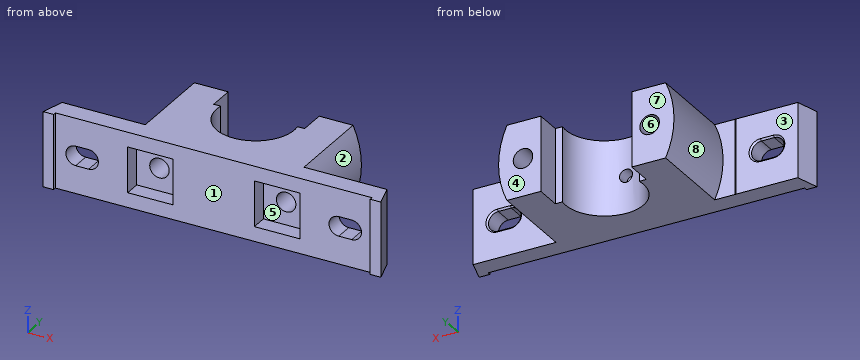
from build123d import *

# Parameters (mm, degrees)
BOSS_EXTRUDE2_DEPTH  = 46
CUT_EXTRUDE1_START   = -52.000000108
CUT_EXTRUDE1_DEPTH   = 36.000000108
CUT_EXTRUDE1_START_2 = 18
CUT_EXTRUDE1_2_DEPTH = 10
CUT_EXTRUDE4_DEPTH   = 126.888839891
CHAMFER1_SIZE        = 1
CUT_EXTRUDE6_DEPTH   = 54
SKETCH7_W            = 28
SKETCH7_H            = 28
CUT_EXTRUDE7_DEPTH   = 10
SKETCH8_R            = 6
CUT_EXTRUDE8_DEPTH   = 127.759615321


with BuildPart() as part:
    # Sketch1 → Boss-Extrude2 (new body)
    with BuildSketch(Plane.XY):
        with BuildLine():
            Line((-28, 20), (-28, 4))
            Line((-28, 4), (-23.664319132, 4))
            ThreePointArc((-23.664319132, 4), (0, -24), (23.664319132, 4))
            Line((23.664319132, 4), (28, 4))
            Line((28, 4), (28, 20))
            Line((28, 20), (54, 20))
            Line((54, 20), (54, -26))
            ThreePointArc((54, -26), (56.343145751, -31.656854249), (62, -34))
            Line((62, -34), (99.985564599, -34))
            Line((99.985564599, -34), (104, -48))
            Line((104, -48), (97.5, -48))
            Line((97.5, -48), (97.5, -46))
            Line((97.5, -46), (-97.5, -46))
            Line((-97.5, -46), (-97.5, -48))
            Line((-97.5, -48), (-104, -48))
            Line((-104, -48), (-99.985564599, -34))
            Line((-99.985564599, -34), (-62, -34))
            ThreePointArc((-62, -34), (-56.343145751, -31.656854249), (-54, -26))
            Line((-54, -26), (-54, 20))
            Line((-54, 20), (-28, 20))
        make_face()
    extrude(amount=BOSS_EXTRUDE2_DEPTH)

    # Cut-Extrude1: read off the stored shape, not the designer's step
    # Cut-Extrude1 outline → Cut-Extrude1 (cut)
    with BuildSketch(Plane(origin=(0, 20, 0), x_dir=(1, 0, 0), z_dir=(0, 1, 0)).offset(CUT_EXTRUDE1_START)):
        with BuildLine():
            add(Edge.make_bspline(
                [(-4, -23), (-4, -21.940981337), (-3.564754015, -20.907732875), (-2.091459192, -19.434771906), (-1.047779124, -19.000600686), (1.043187737, -18.999400631), (2.08248981, -19.42606245), (3.572744195, -20.91546352), (3.999590121, -21.953345573), (4.000409264, -24.043519212), (3.567812098, -25.087662609), (2.094321457, -26.563907402), (1.060428453, -26.999150693), (-1.054011474, -27.000846733), (-2.089559005, -26.5661873), (-3.563043078, -25.094915922), (-4, -24.059018663), (-4, -23)],
                knots=[0, 0, 0, 0, 0.125, 0.125, 0.25, 0.25, 0.375, 0.375, 0.5, 0.5, 0.625, 0.625, 0.75, 0.75, 0.875, 0.875, 1, 1, 1, 1], degree=3))
        make_face()
    extrude(amount=CUT_EXTRUDE1_DEPTH, mode=Mode.SUBTRACT)

    # Cut-Extrude1 2 outline → Cut-Extrude1 2 (add)
    with BuildSketch(Plane.XY.offset(CUT_EXTRUDE1_START_2)):
        with BuildLine():
            Line((5, -31.49528396), (4.000099427, -31.664302326))
            ThreePointArc((4.000099427, -31.664302326), (2.007080448, -31.915928334), (-8.2e-08, -32))
            Line((-8.2e-08, -32), (5, -32.000000108))
            Line((5, -32.000000108), (5, -31.49528396))
        make_face()
        with BuildLine():
            Line((-5, -32.000000108), (-8.2e-08, -32))
            ThreePointArc((-8.2e-08, -32), (-2.00703047, -31.915932528), (-4.000000362, -31.664319071))
            Line((-4.000000362, -31.664319071), (-5, -31.495288265))
            Line((-5, -31.495288265), (-5, -32.000000108))
        make_face()
    extrude(amount=CUT_EXTRUDE1_2_DEPTH)

    # Sketch5 → Cut-Extrude4 (cut, through all)
    with BuildSketch(Plane(origin=(0, -34, 0), x_dir=(1, 0, 0), z_dir=(0, 1, 0))):
        with BuildLine():
            Line((77, -17), (85, -17))
            ThreePointArc((85, -17), (91, -23), (85, -29))
            Line((85, -29), (77, -29))
            ThreePointArc((77, -29), (71, -23), (77, -17))
        make_face()
        with BuildLine():
            Line((-77, -17), (-85, -17))
            ThreePointArc((-85, -17), (-91, -23), (-85, -29))
            Line((-85, -29), (-77, -29))
            ThreePointArc((-77, -29), (-71, -23), (-77, -17))
        make_face()
    extrude(amount=-CUT_EXTRUDE4_DEPTH, mode=Mode.SUBTRACT)

    # Chamfer1
    chamfer1_edges = [part.edges().sort_by_distance(p)[0] for p in [
        (71, -34, 23),
        (81, -34, 29),
        (91, -34, 23),
        (81, -34, 17),
        (-71, -34, 23),
        (-81, -34, 17),
        (-91, -34, 23),
        (-81, -34, 29),
    ]]
    chamfer(chamfer1_edges, length=CHAMFER1_SIZE)

    # Sketch6 → Cut-Extrude6 (cut)
    with BuildSketch(Plane(origin=(0, 20, 0), x_dir=(1, 0, 0), z_dir=(0, 1, 0))):
        with BuildLine():
            Line((54, -46), (48.856934001, -46))
            ThreePointArc((48.856934001, -46), (54, -23), (48.856934001, 0))
            Line((48.856934001, 0), (54, 0))
            Line((54, 0), (63.209098635, 0))
            Line((63.209098635, 0), (63.209098635, -46))
            Line((63.209098635, -46), (54, -46))
        make_face()
        with BuildLine():
            Line((-48.856934001, -46), (-54, -46))
            Line((-54, -46), (-61.379097466, -46))
            Line((-61.379097466, -46), (-61.379097466, 0))
            Line((-61.379097466, 0), (-54, 0))
            Line((-54, 0), (-48.856934001, 0))
            ThreePointArc((-48.856934001, 0), (-54, -23), (-48.856934001, -46))
        make_face()
    extrude(amount=-CUT_EXTRUDE6_DEPTH, mode=Mode.SUBTRACT)

    # Sketch7 → Cut-Extrude7 (cut)
    with BuildSketch(Plane.XZ.offset(46)):
        with Locations((-39, 23)):
            Rectangle(SKETCH7_W, SKETCH7_H)
        with Locations((39, 23)):
            Rectangle(SKETCH7_W, SKETCH7_H)
    extrude(amount=-CUT_EXTRUDE7_DEPTH, mode=Mode.SUBTRACT)

    # Sketch8 → Cut-Extrude8 (cut, through all)
    with BuildSketch(Plane.XZ.offset(36)):
        with Locations((-39, 23)):
            Circle(SKETCH8_R)
        with Locations((39, 23)):
            Circle(SKETCH8_R)
    extrude(amount=-CUT_EXTRUDE8_DEPTH, mode=Mode.SUBTRACT)


solid = part.part
Model file for the job. Use its own axes, mm. Face numbers are marked on the shaded views. A direction names the side the tool comes from. Give positions to 0.01 mm unless a question says otherwise; leave off trailing zeros. Order: outer loops, then holes, each group sorted by start corner. A loop starts at its lowest first (then second) coordinate and runs counter-clockwise, first axis right, second up. Notation, with made-up numbers: M -35.75,77.25 L -25.75,77.25 A18 ccw -25.75,86.25 Z; hole C -26,-14 d5. An arc over 180 degrees is marked long. Put each result on its own line as item: value. Start each with the question number.
(1) Band-saw the part on C-C on y = -19. Give the cut face in (x, z), then the cut area to 3 significant figures.
(2) Band-saw the part on A-A on y = 0. Give the cut face in (x, z), then the cut area to 3 significant figures.
(3) Drill centre lines: L1, parallel to Z at x = -39, y = 2.5; L2, parallel to X at y = -15.5, z = 18; L3, parallel to X at y = 16.5, z = 8. Where is each one in solid material? Low to high. Write a range as [from, to].
(4) Band-saw the part on B-B on x = 39. Give the cut face in (y, z), then the cut area to 3 significant figures.
(5) Tool access for the marked faces 1, 2, 3, 4 and 5: list every direction of +Z, -Z, +X, -X, +Y, -Y with a clear straight run to the whole face (end or side of a thin tool).
(6) Pin check, flat tips, straight feed: pin 1 Ø1 at (y, z) = (-2.5, 11.5) entering from +X; pin 2 Ø12 at (y, z) = (-3.5, 16) entering from +X; pin 3 Ø2 at (x, z) = (25, 25) entering from +Y. Stop position of each tip, or through.
(7) Band-saw the part on D-D on x = -17. Give the cut face in (y, z).
(8) Pull direction X, two halves, no side cores. Call the marked faces 6, 7 and 8: released by +X, released by -X, zero draft, split by the parting line, or undercut.
Results below:
1. outline: M -48.86,0 L -14.66,0 L -14.66,46 L -48.86,46 A54 ccw Z; M 14.66,0 L 48.86,0 A54 ccw 48.86,46 L 14.66,46 Z; hole C -39,23 d12; hole C 39,23 d12
1. area: 3,240 mm2
2. outline: M -48.86,0 L -24,0 L -24,46 L -48.86,46 A54 ccw Z; M 24,0 L 48.86,0 A54 ccw 48.86,46 L 24,46 Z; hole C -39,23 d12; hole C 39,23 d12
2. area: 2,380 mm2
3. L1: z = [0, 17], [29, 46]
3. L2: x = [-53.77, -42.32], [-35.68, -18.32], [18.32, 35.68], [42.32, 53.77]
3. L3: x = [-51.87, -28], [28, 51.87]
4. outline: M -46,0 L 20,0 L 20,17 L -36,17 L -36,9 L -46,9 Z; M -46,37 L -36,37 L -36,29 L 20,29 L 20,46 L -46,46 Z
4. area: 2,080 mm2
5. face 1: +Z, -Z, -Y
5. face 2: +X, +Y
5. face 3: +Z, -Z, -X, +Y
5. face 4: +Z, -Z, +X, -X, +Y
5. face 5: -Y
6. pin 1: stops at x = 52.87
6. pin 2: stops at x = 53.99
6. pin 3: stops at y = 4
7. outline: M -46,0 L -16.94,0 L -16.94,46 L -46,46 Z
8. face 6: undercut
8. face 7: zero draft
8. face 8: released by -X
